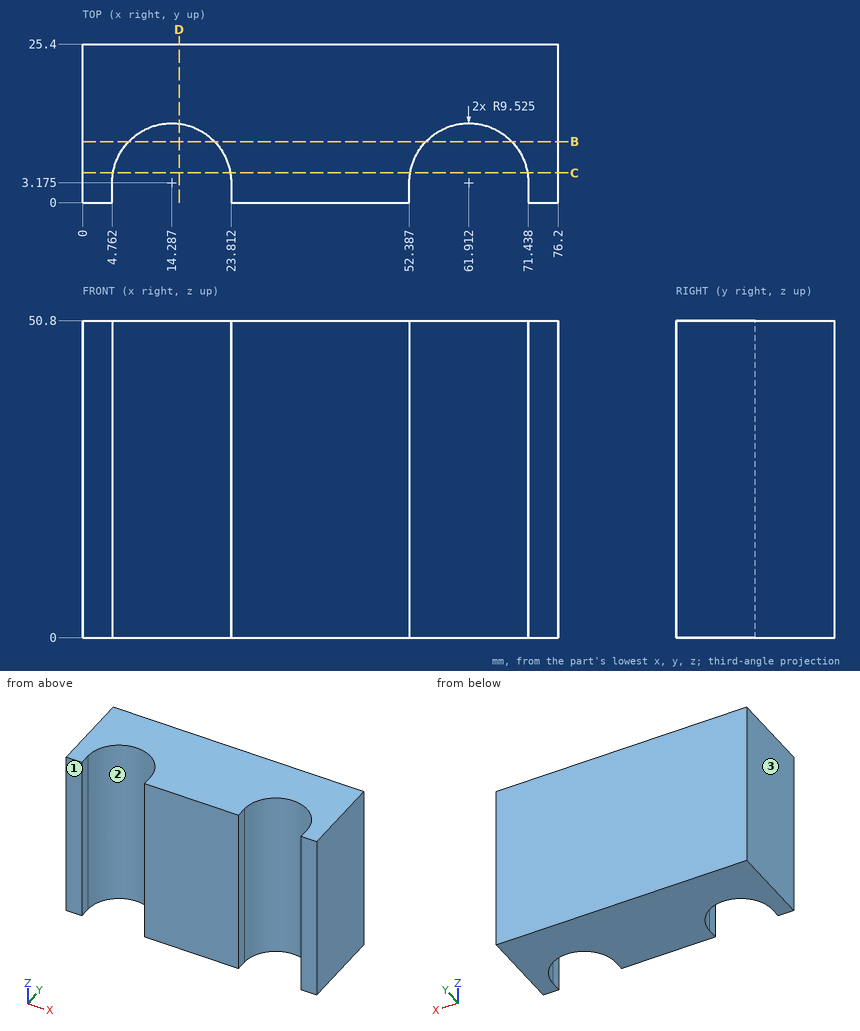
Geometry check sheet. Reference: drawing and pictorial views, mm from the part's lowest x, y, z. Give positions to 0.01 mm unless a question says otherwise; leave off trailing zeros. Order: outer loops, then holes, each group sorted by start corner. A loop starts at its lowest first (then second) coordinate and runs counter-clockwise, first axis right, second up. Notation, with made-up numbers: M 61.5,52 L 71.5,52 A24 ccw 71.5,66 Z; hole C 87,65 d1. An arc over 180 degrees is marked long. Answer as CSV lines item,"result". Start each with the question number.
Item 1: Mould release check, pull along X, two halves, no side actions. Record for the marked faces 1, 2 and 3: +X half, -X half, draft (parallel to the pull), parting line (faces both ways), or undercut.
Item 2: Thickness scan on line 1 (X direction, y = 2, z = 8); line 2 (X direction, y = 10.5, z = 31) (1 decimal); line 3 (Y direction, x = 54, z = 26) (1 decimal). Record the ranges inside material, lowest first. Write a range as [from, to].
Item 3: Cross-section at C-C on y = 4.75. Enter the section's corners in (x, z).
Item 4: Cross-section at D-D on x = 15.5. Enter the section's corners in (y, z), plus the area to 3 significant figures.
Item 5: Cross-section at B-B on y = 9.75. Enter the section's corners in (x, z) (1 decimal).
Established:
1,face 1,"draft"
1,face 2,"undercut"
1,face 3,"-X half"
2,line 1,"x = [0, 4.76], [23.81, 52.39], [71.44, 76.2]"
2,line 2,"x = [0, 8.2], [20.4, 55.8], [68, 76.2]"
2,line 3,"y = [8.5, 25.4]"
3,outline,"M 0,0 L 4.89,0 L 4.89,50.8 L 0,50.8 Z; M 23.68,0 L 52.52,0 L 52.52,50.8 L 23.68,50.8 Z; M 71.31,0 L 76.2,0 L 76.2,50.8 L 71.31,50.8 Z"
4,outline,"M 12.62,0 L 25.4,0 L 25.4,50.8 L 12.62,50.8 Z"
4,area,"649 mm^2"
5,outline,"M 0,0 L 7.4,0 L 7.4,50.8 L 0,50.8 Z; M 21.2,0 L 55,0 L 55,50.8 L 21.2,50.8 Z; M 68.8,0 L 76.2,0 L 76.2,50.8 L 68.8,50.8 Z"
